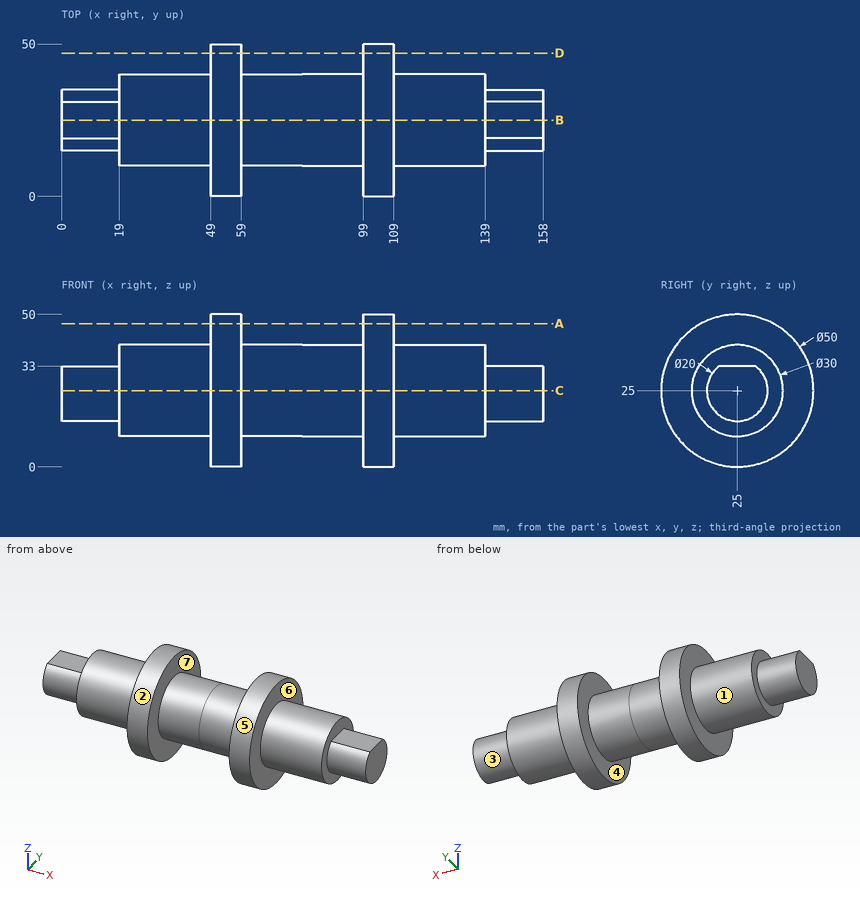
The figure shows three views and two pictorial views of one solid part (mm, origin at its lowest corner). Answer the questions. A direction names the side the tool comes from. Round coordinates to 2 decimals unless told otherwise and drop trailing zeros. Write each loop counter-clockwise with the first axis right and the second up, starting at its lowest first coordinate (ties: lowest second). Pieces come first, ordered by that corner, then holes. Notation, with made-up numbers: (4, 78.5) - (43, 78.5) arc R33 ccw to (43, 108.5) - close; hole circle Ø1 at (52.25, -3.5). An arc over 180 degrees is marked (long way). Answer in a Markdown table with one row per item. Add a question column.
1. For the marked faces 1, 2 and 3, determine the directions among +Z, -Z, +X, -X, +Y, -Y from which every point of the face is accessible in a straight line to the end or side of a thin tool.
2. A cutting plane is placed at B-B, the plane y = 25. Determine the outline of the cut face in (x, z).
3. A cutting plane is placed at A-A, the plane z = 47. Determine the outline of the cut face in (x, y).
4. Given pin 1 (5 mm diameter, centred on x = 81, z = 30.5, fed in from -Y); pin 2 (1.5 mm diameter, centred on x = 124, y = 38, fed in from +Z); pin 3 (3 mm diameter, centred on x = 41.5, z = 23.5, fed in from +Y), each flat-ended and moving along its own axis, determine where each tip first touches the part or whether it passes through.
5. The mould has two halves that part along X. Classify the marked faces 4, 5, 6 and 7: +X half, -X half, draft (parallel to the pull), parting line (faces both ways), or undercut.
6. A cutting plane is placed at C-C, the plane z = 25. Determine the outline of the cut face in (x, y), and give its area (3 significant figures).
7. Find the intervals of material crossed by line 1 along X through (y, z) = (9.5, 18.5); line 2 along X through (y, z) = (17, 35); line 3 along Y through (x, z) = (85, 26), in increasing order. Write a range as from..to.
Worked out:
| question | item | result |
|---|---|---|
| 1 | face 1 | -X |
| 1 | face 2 | +X, -X |
| 1 | face 3 | +X |
| 2 | outline | (0, 15) - (19, 15) - (19, 10) - (49, 10) - (49, 0) - (59, 0) - (59, 10) - (99, 10) - (99, 0) - (109, 0) - (109, 10) - (139, 10) - (139, 15) - (158, 15) - (158, 33) - (139, 33) - (139, 40) - (109, 40) - (109, 50) - (99, 50) - (99, 40) - (59, 40) - (59, 50) - (49, 50) - (49, 40) - (19, 40) - (19, 33) - (0, 33) - close |
| 3 | outline | (49, 13.13) - (59, 13.13) - (59, 36.87) - (49, 36.87) - close; (99, 13.13) - (109, 13.13) - (109, 36.87) - (99, 36.87) - close |
| 4 | pin 1 | y = 10.3 |
| 4 | pin 2 | z = 33.66 |
| 4 | pin 3 | y = 40 |
| 5 | face 4 | undercut |
| 5 | face 5 | draft |
| 5 | face 6 | +X half |
| 5 | face 7 | undercut |
| 6 | outline | (0, 15) - (19, 15) - (19, 10) - (49, 10) - (49, 0) - (59, 0) - (59, 10) - (99, 10) - (99, 0) - (109, 0) - (109, 10) - (139, 10) - (139, 15) - (158, 15) - (158, 35) - (139, 35) - (139, 40) - (109, 40) - (109, 50) - (99, 50) - (99, 40) - (59, 40) - (59, 50) - (49, 50) - (49, 40) - (19, 40) - (19, 35) - (0, 35) - close |
| 6 | area | 4,760 mm^2 |
| 7 | line 1 | 49..59, 99..109 |
| 7 | line 2 | 19..139 |
| 7 | line 3 | 10.03..39.97 |
